```python
from build123d import *

# Parameters (mm, degrees)
F0_W      = 53
F0_H      = 53
F1_DEPTH  = 14
F0_H_2    = 49
F2_DEPTH  = 14
F3_T      = -2.5
F5_DEPTH  = 53
F6_DEPTH  = 53
F7_T      = -2.5
F9_R      = 18
F10_R     = 5
F11_T     = -2
F12_DEPTH = 7.2
F14_R     = 25


with BuildPart() as f1:
    # F0 (on Top) → F1 (new body)
    with BuildSketch(Plane.XY):
        with Locations((0, -24.5)):
            Rectangle(F0_W, F0_H)
    extrude(amount=F1_DEPTH)

    # F3
    f3_openings = [f1.faces().sort_by_distance(p)[0] for p in [
        (0, -24.5, 14),
    ]]
    offset(amount=F3_T, openings=f3_openings)


with BuildPart() as f2:
    # F0 (on Top) → F2 (new body)
    with BuildSketch(Plane.XY):
        with Locations((0, 26.5)):
            Rectangle(F0_W, F0_H_2)
    extrude(amount=F2_DEPTH)


with BuildPart() as f5:
    # F4 (on face) → F5 (new body, through all)
    with BuildSketch(Plane.YZ.offset(26.5)):
        Polygon((-16, 36.5), (2, 14), (51, 14), (51, 22.5), (0.4205387023, 64.94120732), align=None)
    extrude(amount=-F5_DEPTH)

    # F9
    f9_edges = [f5.edges().sort_by_distance(p)[0] for p in [
        (0, 51, 22.5),
    ]]
    fillet(f9_edges, radius=F9_R)

    # F10
    f10_edges = [f5.edges().sort_by_distance(p)[0] for p in [
        (0, 0.420539, 64.941207),
    ]]
    fillet(f10_edges, radius=F10_R)

    # F11
    f11_openings = [f5.faces().sort_by_distance(p)[0] for p in [
        (26.5, 14.357834, 32.967777),
    ]]
    offset(amount=F11_T, openings=f11_openings)

    # F8 (on face) → F12 (cut)
    with BuildSketch(Plane(origin=(0, -27.8049636191, 16.0532032303), x_dir=(1, 0, 0), z_dir=(0, -0.8660254038, 0.5))):
        with BuildLine():
            Line((17, 52.0304659404), (-17, 52.0304659404))
            ThreePointArc((-17, 52.0304659404), (-20.5355339059, 50.5659998464), (-22, 47.0304659404))
            Line((-22, 47.0304659404), (-22, 33.0304659404))
            ThreePointArc((-22, 33.0304659404), (-20.5355339059, 29.4949320345), (-17, 28.0304659404))
            Line((-17, 28.0304659404), (17, 28.0304659404))
            ThreePointArc((17, 28.0304659404), (20.5355339059, 29.4949320345), (22, 33.0304659404))
            Line((22, 33.0304659404), (22, 47.0304659404))
            ThreePointArc((22, 47.0304659404), (20.5355339059, 50.5659998464), (17, 52.0304659404))
        make_face()
    extrude(amount=-F12_DEPTH, mode=Mode.SUBTRACT)


with BuildPart() as f6:
    # F4 (on face) → F6 (new body, through all)
    with BuildSketch(Plane.YZ.offset(26.5)):
        Polygon((-16, 14), (2, 14), (-16, 36.5), align=None)
        Polygon((-16, 36.5), (-28.9903810568, 14), (-16, 14), align=None)
    extrude(amount=-F6_DEPTH)

    # F7
    f7_openings = [f6.faces().sort_by_distance(p)[0] for p in [
        (0, -22.495191, 25.25),
        (0, -13.495191, 14),
    ]]
    offset(amount=F7_T, openings=f7_openings)

    # F13: union F5, F2, F1
    add(f5.part)
    add(f2.part)
    add(f1.part)

    # F14
    f14_edges = [f6.edges().sort_by_distance(p)[0] for p in [
        (25.25, -28.990381, 14),
        (-25.25, -28.990381, 14),
    ]]
    fillet(f14_edges, radius=F14_R)


solid = f6.part
```
Here's how the part is built. I have some questions about the finished solid (model axes, mm). A direction names the side the tool comes from. Coordinates: 2 decimals unless noted, no trailing zeros. Order: outer loops, then holes, each group sorted by start corner. A loop starts at its lowest first (then second) coordinate and runs counter-clockwise, first axis right, second up. Notation, with made-up numbers: (-6.5, 25.5) - (24.5, 25.5) arc R20 cw to (24.5, 34.5) - close; hole circle Ø10 at (4.5, 45.5). An arc over 180 degrees is marked (long way). One line per question, with ' | ' between items. Start each with the question number.
1. If we section it at D-D (y = 31): Write out the boundary of the cut face in (x, z), and give its area (3 significant figures).
2. If we section it at C-C (z = 6): Write out the boundary of the cut face in (x, y), and give its area (3 significant figures).
3. If we section it at A-A (z = 51.5): Write out the boundary of the cut face in (x, y).
4. If we mould it in two halves opening along X, with no side actions, what happens to faces 6 (the flat face through (1, 26, 16)), 7 (the flat face through (26.5, 0, 15)), 8 (the flat face through (0, -48.5, 8))? For each: released by +X, released by -X, zero draft, split by the parting line, or undercut.
5. Please list where these lines run through material, in increasing order: line 1 along Y through (x, z) = (10.5, 5); line 2 along Z through (x, y) = (-14, -45.5); line 3 along Z through (x, y) = (10, 5). Write a range as [from, to].
6. Which directions (+Z, -Z, +X, -X, +Y, -Y) give clear straight access to the entire face, cutting with the end or side of a thin tool? Please do faces 1 (the flat face through (0, -0.5, 8)), 2 (the flat face through (0.34, -9.16, 23.95)), 3 (the flat face through (1.36, 23.77, 42.74)), 4 (the cylindrical face through (-0.37, 49.36, 21.61)), 5 (the cylindrical face through (20.5, -12.22, 41.07)).
7. I'm going to push flat-ended pins straight in: pin 1 Ø2 at (x, y) = (-20, 35.5) entering from +Z; pin 2 Ø8.5 at (x, y) = (-9, -46) entering from +Z; pin 3 Ø2 at (x, z) = (-14, 44) entering from +Y. Where does each tip first touch, or does it pass through?
8. If we section it at B-B (x = -5): Write out the boundary of the cut face in (y, z), and give its area (3 significant figures).
Model answer:
1) outline: (-26.5, 0) - (26.5, 0) - (26.5, 16) - (-24.5, 16) - (-24.5, 36.67) - (26.5, 36.67) - (26.5, 39.28) - (-26.5, 39.28) - close | area: 1,030 mm²
2) outline: (-26.5, -51) - (26.5, -51) - (26.5, 51) - (-26.5, 51) - close; hole (-24, -48.5) - (24, -48.5) - (24, -0.5) - (-24, -0.5) - close | area: 3,100 mm²
3) outline: (-26.5, -7.34) - (-22, -7.34) - (-22, -5.03) - (-24.5, -5.03) - (-24.5, 13.33) - (26.5, 13.33) - (26.5, 16.44) - (-26.5, 16.44) - close; (22, -7.34) - (26.5, -7.34) - (26.5, -5.03) - (22, -5.03) - close
4) face 6: zero draft | face 7: released by +X | face 8: undercut
5) line 1: y = [-51, -48.5], [-0.5, 51] | line 2: z = [0, 2.5] | line 3: z = [0, 16], [58.49, 61.1]
6) face 1: none | face 2: -Y | face 3: +X | face 4: +Z, +X, -X, +Y | face 5: +Z
7) pin 1: stops at z = 36.35 | pin 2: stops at z = 14 | pin 3: stops at y = 26.57
8) outline: (-51, 0) - (51, 0) - (51, 14.11) arc R18 ccw to (44.57, 27.9) - (4.99, 61.11) arc R5 ccw to (-1.58, 60.99) - (0.31, 59.9) arc R3 cw to (3.7, 59.58) - (43.28, 26.36) arc R16 cw to (48.89, 16) - (2.96, 16) - (-13.59, 36.68) - (-12.06, 39.33) - (-13.79, 40.33) - (-17.34, 34.18) - (-1.2, 14) - (-0.5, 14) - (-0.5, 2.5) - (-48.5, 2.5) - (-48.5, 14) - (-51, 14) - close | area: 1,240 mm²
